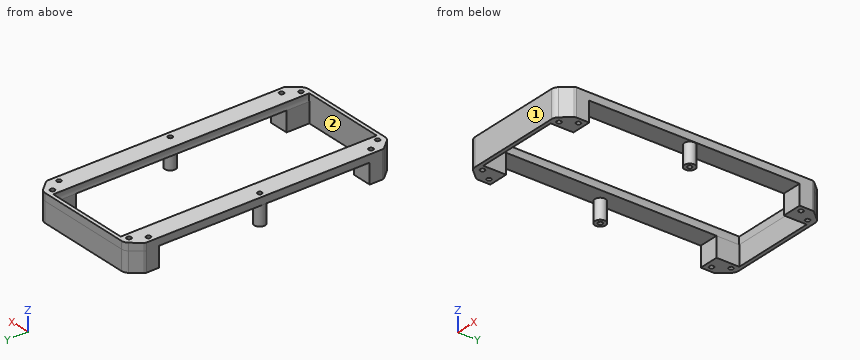
```python
from build123d import *

# Parameters (mm, degrees)
SKETCH066_R     = 7.357041
SKETCH066_R_2   = 3
EXTRUDE_DEPTH   = 26.75
SKETCH065_R     = 3
SKETCH065_W     = 114.5
SKETCH065_H     = 345
PAD035_DEPTH    = 10
POCKET035_DEPTH = 345


with BuildPart() as body082:
    # Sketch066 → Extrude (new body)
    with BuildSketch(Plane.XY):
        with Locations((-76, 0)):
            Circle(SKETCH066_R)
        with Locations((-76, 0)):
            Circle(SKETCH066_R_2, mode=Mode.SUBTRACT)
        with Locations((76, 0)):
            Circle(SKETCH066_R)
        with Locations((76, 0)):
            Circle(SKETCH066_R_2, mode=Mode.SUBTRACT)
        with BuildLine():
            ThreePointArc((-83.039601, 161.795278), (-83.752226, 160.581048), (-84, 159.195119))
            Line((-84, 141.77214), (-84, 159.195119))
            Line((-84, 141.77214), (-57.25, 141.77214))
            Line((-57.25, 141.77214), (-57.25, 172.5))
            Line((-57.25, 172.5), (57.25, 172.5))
            Line((57.25, 141.77214), (57.25, 172.5))
            Line((84, 141.77214), (57.25, 141.77214))
            Line((84, 141.77214), (84, 159.195119))
            ThreePointArc((84, 159.195119), (83.752226, 160.581048), (83.039601, 161.795278))
            Line((72.599002, 174.000398), (83.039601, 161.795278))
            ThreePointArc((72.599002, 174.000398), (69.183062, 176.583061), (65, 177.5))
            Line((-65, 177.5), (65, 177.5))
            ThreePointArc((-65, 177.5), (-69.183062, 176.583061), (-72.599002, 174.000398))
            Line((-72.599002, 174.000398), (-83.039601, 161.795278))
        make_face()
        with Locations((-65, 167.5)):
            Circle(SKETCH066_R_2, mode=Mode.SUBTRACT)
        with Locations((-76, 150)):
            Circle(SKETCH066_R_2, mode=Mode.SUBTRACT)
        with Locations((65, 167.5)):
            Circle(SKETCH066_R_2, mode=Mode.SUBTRACT)
        with Locations((76, 150)):
            Circle(SKETCH066_R_2, mode=Mode.SUBTRACT)
        with BuildLine():
            ThreePointArc((-84, -159.195119), (-83.752226, -160.581048), (-83.039601, -161.795278))
            Line((-72.599002, -174.000398), (-83.039601, -161.795278))
            ThreePointArc((-72.599002, -174.000398), (-69.183062, -176.583061), (-65, -177.5))
            Line((-65, -177.5), (65, -177.5))
            ThreePointArc((65, -177.5), (69.183062, -176.583061), (72.599002, -174.000398))
            Line((72.599002, -174.000398), (83.039601, -161.795278))
            ThreePointArc((83.039601, -161.795278), (83.752226, -160.581048), (84, -159.195119))
            Line((84, -141.77214), (84, -159.195119))
            Line((84, -141.77214), (57.25, -141.77214))
            Line((57.25, -141.77214), (57.25, -172.5))
            Line((-57.25, -172.5), (57.25, -172.5))
            Line((-57.25, -141.77214), (-57.25, -172.5))
            Line((-84, -141.77214), (-57.25, -141.77214))
            Line((-84, -141.77214), (-84, -159.195119))
        make_face()
        with Locations((-65, -167.5)):
            Circle(SKETCH066_R_2, mode=Mode.SUBTRACT)
        with Locations((-76, -150)):
            Circle(SKETCH066_R_2, mode=Mode.SUBTRACT)
        with Locations((65, -167.5)):
            Circle(SKETCH066_R_2, mode=Mode.SUBTRACT)
        with Locations((76, -150)):
            Circle(SKETCH066_R_2, mode=Mode.SUBTRACT)
    extrude(amount=-EXTRUDE_DEPTH)


with BuildPart() as body081:
    # Sketch065 → Pad035 (new body)
    with BuildSketch(Plane.XY):
        with BuildLine():
            Line((84, -33.872292), (84, 33.872292))
            Line((84, 159.195119), (84, 33.872292))
            ThreePointArc((84, 159.195119), (83.752226, 160.581048), (83.039601, 161.795278))
            Line((72.599002, 174.000398), (83.039601, 161.795278))
            ThreePointArc((72.599002, 174.000398), (69.183062, 176.583061), (65, 177.5))
            Line((-65, 177.5), (65, 177.5))
            ThreePointArc((-65, 177.5), (-69.183062, 176.583061), (-72.599002, 174.000398))
            Line((-83.039601, 161.795278), (-72.599002, 174.000398))
            ThreePointArc((-83.039601, 161.795278), (-83.752226, 160.581048), (-84, 159.195119))
            Line((-84, 33.872292), (-84, 159.195119))
            Line((-84, 33.872292), (-84, -33.872292))
            Line((-84, -33.872292), (-84, -159.195119))
            ThreePointArc((-84, -159.195119), (-83.752226, -160.581048), (-83.039601, -161.795278))
            Line((-83.039601, -161.795278), (-72.599002, -174.000398))
            ThreePointArc((-72.599002, -174.000398), (-69.183062, -176.583061), (-65, -177.5))
            Line((-65, -177.5), (65, -177.5))
            ThreePointArc((65, -177.5), (69.183062, -176.583061), (72.599002, -174.000398))
            Line((72.599002, -174.000398), (83.039601, -161.795278))
            ThreePointArc((83.039601, -161.795278), (83.752226, -160.581048), (84, -159.195119))
            Line((84, -159.195119), (84, -33.872292))
        make_face()
        with Locations((-76, 150)):
            Circle(SKETCH065_R, mode=Mode.SUBTRACT)
        with Locations((76, 150)):
            Circle(SKETCH065_R, mode=Mode.SUBTRACT)
        with Locations((-76, -150)):
            Circle(SKETCH065_R, mode=Mode.SUBTRACT)
        with Locations((76, -150)):
            Circle(SKETCH065_R, mode=Mode.SUBTRACT)
        with Locations((76, 0)):
            Circle(SKETCH065_R, mode=Mode.SUBTRACT)
        with Locations((-76, 0)):
            Circle(SKETCH065_R, mode=Mode.SUBTRACT)
        with Locations((-65, 167.5)):
            Circle(SKETCH065_R, mode=Mode.SUBTRACT)
        with Locations((65, 167.5)):
            Circle(SKETCH065_R, mode=Mode.SUBTRACT)
        with Locations((-65, -167.5)):
            Circle(SKETCH065_R, mode=Mode.SUBTRACT)
        with Locations((65, -167.5)):
            Circle(SKETCH065_R, mode=Mode.SUBTRACT)
        Rectangle(SKETCH065_W, SKETCH065_H, mode=Mode.SUBTRACT)
    extrude(amount=PAD035_DEPTH)

    # Sketch068 (on Face21 of Pad035) → Pocket035 (cut)
    with BuildSketch(Plane(origin=(0, -172.5, 0), x_dir=(-1, 0, 0), z_dir=(0, 1, 0))):
        with BuildLine():
            ThreePointArc((-57.25, 10), (-57.885083, 5), (-57.25, 0))
            Line((-57.25, 10), (-57.25, 0))
        make_face()
        with BuildLine():
            ThreePointArc((57.25, 0), (57.885083, 5), (57.25, 10))
            Line((57.25, 10), (57.25, 0))
        make_face()
    extrude(amount=POCKET035_DEPTH, mode=Mode.SUBTRACT)

    # Boolean006: union Body082
    add(body082.part)


solid = body081.part
```
Input: part model. Units: mm. Frame: model coordinates. Face numbers are marked on the shaded views. Coordinates: 2 decimals unless noted, no trailing zeros. Loops run counter-clockwise (first coordinate to the right, second up) from the corner with the lowest first, then second, coordinate; pieces in that order, holes last.
Q1. Section C-C, the plane z = 4. Give the number of separate pieces and of enclosed holes in the cut face, and give its area (3 significant figures).
Results are:
separate pieces: 1
enclosed holes: 11
area: 18,900 mm2
Q2. Mould query, pull axis Y, two halves, no side actions, for the marked faces 1 and 2. Classes: +Y half, -Y half, draft (parallel to the pull), parting line (faces both ways), or undercut.
Results are:
face 1: -Y half
face 2: undercut
Q3. Section A-A, the plane y = -47.5. Return the cut outline in (x, z), and give its area (3 significant figures).
Results are:
outline: (-84, 0) - (-57.25, 0) arc R20 cw to (-57.25, 10) - (-84, 10) - close; (57.25, 0) - (84, 0) - (84, 10) - (57.25, 10) arc R20 cw to start
area: 527 mm2
Q4. Section B-B, the plane x = 40.5. Return the cut outline in (y, z).
Results are:
outline: (-177.5, -26.75) - (-172.5, -26.75) - (-172.5, 10) - (-177.5, 10) - close; (172.5, -26.75) - (177.5, -26.75) - (177.5, 10) - (172.5, 10) - close
Q5. Contact query for a flat-ended pin moving along its axis: pin 1 (6 mm diameter, centred on x = 54.5, y = -109.5, fed in from -Z). Output: stop coordinate, or through.
Results are:
pin 1: stops at z = 0
Q6. Line query: line 1 along X through (y, z) = (-150, -5); line 2 along X through (y, z) = (-150, 5.25); line 3 along Y through (x, z) = (14.5, -3). Output: solid intervals per line, ascending.
Results are:
line 1: x = -84 to -79, -73 to -57.25, 57.25 to 73, 79 to 84
line 2: x = -84 to -79, -73 to -57.88, 57.88 to 73, 79 to 84
line 3: y = -177.5 to -172.5, 172.5 to 177.5
